The listing builds one solid part. Answer for the finished solid, in the listing's coordinates (mm). Round coordinates to 2 decimals unless told otherwise and drop trailing zeros. Loops run counter-clockwise (first coordinate to the right, second up) from the corner with the lowest first, then second, coordinate; pieces in that order, holes last. Notation, with made-up numbers: (78, 40.25) - (86, 40.25) arc R21 cw to (86, 79.25) - close; hole circle Ø6 at (24.25, 50.25). An arc over 180 degrees is marked (long way). One line per item, written item: value.
Autodesk Inventor part; units mm, degrees
ref_plane "YZ Plane" through (0, 0, 0) normal (1, 0, 0) x (0, 1, 0)
ref_plane "XZ Plane" through (0, 0, 0) normal (0, 1, 0) x (-1, 0, 0)
ref_plane "XY Plane" through (0, 0, 0) normal (0, 0, 1) x (1, 0, 0)
sketch "Sketch1" plane through (0, 0, 0) normal (0, 1, 0) x (-1, 0, 0)
  line L0 (-7.5, 12.5) -> (7.5, 12.5)
  line L1 (7.5, 12.5) -> (7.5, -12.5)
  line L2 (7.5, -12.5) -> (-7.5, -12.5)
  line L3 (-7.5, -12.5) -> (-7.5, 12.5)
  line L4 (-7.5, 12.5) -> (7.5, -12.5) construction
  line L5 (7.5, 12.5) -> (4.96, 12.5)
  line L6 (-7.5, 12.5) -> (-5.5, 12.5)
  circle A0 centre (-5.5, 10.5) radius 1.5
  line L7 (-7.5, -12.5) -> (-7.5, -10.5)
  circle A1 centre (-5.5, -10.5) radius 1.5
  point P0 (0, 0)
  dimension "d0" = 15
  dimension "d1" = 25
  dimension "d9" = 2
  dimension "d11" = 3
  dimension "d12" = 2
  dimension "d14" = 3
extrude "Extrusion1" add sketch "Sketch1" along normal blind 1
properties part number "Compass"
1) A cutting plane is placed at C-C on y = 0.2. Give the vertices of the cut face in (x, z), and give its area (3 significant figures).
Final values:
outline: (-7.5, -12.5) - (7.5, -12.5) - (7.5, 12.5) - (-7.5, 12.5) - close; hole circle Ø3 at (5.5, -10.5); hole circle Ø3 at (5.5, 10.5)
area: 361 mm2
2) A cutting plane is placed at B-B on x = 5.5. Give the vertices of the cut face in (y, z), and give its area (3 significant figures).
Final values:
outline: (0, -12.5) - (1, -12.5) - (1, -12) - (0, -12) - close; (0, -9) - (1, -9) - (1, 9) - (0, 9) - close; (0, 12) - (1, 12) - (1, 12.5) - (0, 12.5) - close
area: 19.0 mm2
3) For a pull along Z with two mould halves and no side action, classify faces 1 (the flat face through (0.1, 0.5, 12.5)), 2 (the cylindrical face through (6.7, 0.5, -9.6)), 3 (the cylindrical face through (6.7, 0.5, 11.4)), 4 (the flat face through (0, 0, 0)) as released by +Z, released by -Z, zero draft, split by the parting line, or undercut.
Final values:
face 1: released by +Z
face 2: undercut
face 3: undercut
face 4: zero draft
4) Consider L1, parallel to Z at x = 5.5, y = 0.4; L2, parallel to X at y = 0.15, z = -9.5; L3, parallel to X at y = 0.8, z = 9.75. Determine where each line is inside the solid, lowest interval first.
Final values:
L1: -12.5 to -12, -9 to 9, 12 to 12.5
L2: -7.5 to 4.38, 6.62 to 7.5
L3: -7.5 to 4.2, 6.8 to 7.5
5) A cutting plane is placed at A-A on z = -10.5. Give the vertices of the cut face in (x, y), and give its area (3 significant figures).
Final values:
outline: (-7.5, 0) - (4, 0) - (4, 1) - (-7.5, 1) - close; (7, 0) - (7.5, 0) - (7.5, 1) - (7, 1) - close
area: 12.0 mm2
6) This flat-tipped pin is pushed along its axis until it touches: pin 1 Ø2 at (x, z) = (4.5, -0.5) entering from -Y. Where does it stop, or does it pass through?
Final values:
pin 1: y = 0
